Input: dimensioned drawing with shaded views. Units: mm. Origin: part minimum x, y, z. A direction names the side the tool comes from. Give positions to 0.01 mm unless a question says otherwise; leave off trailing zeros. Write each loop counter-clockwise with the first axis right and the second up, starting at its lowest first coordinate (ties: lowest second). Pieces come first, ordered by that corner, then holes. Notation, with made-up numbers: M 41,-34.5 L 53,-34.5 A25 cw 53,-4.5 Z; hole C 40.5,-34 d11. An arc over 180 degrees is marked long. Answer as a JSON object with one key per item and string values.
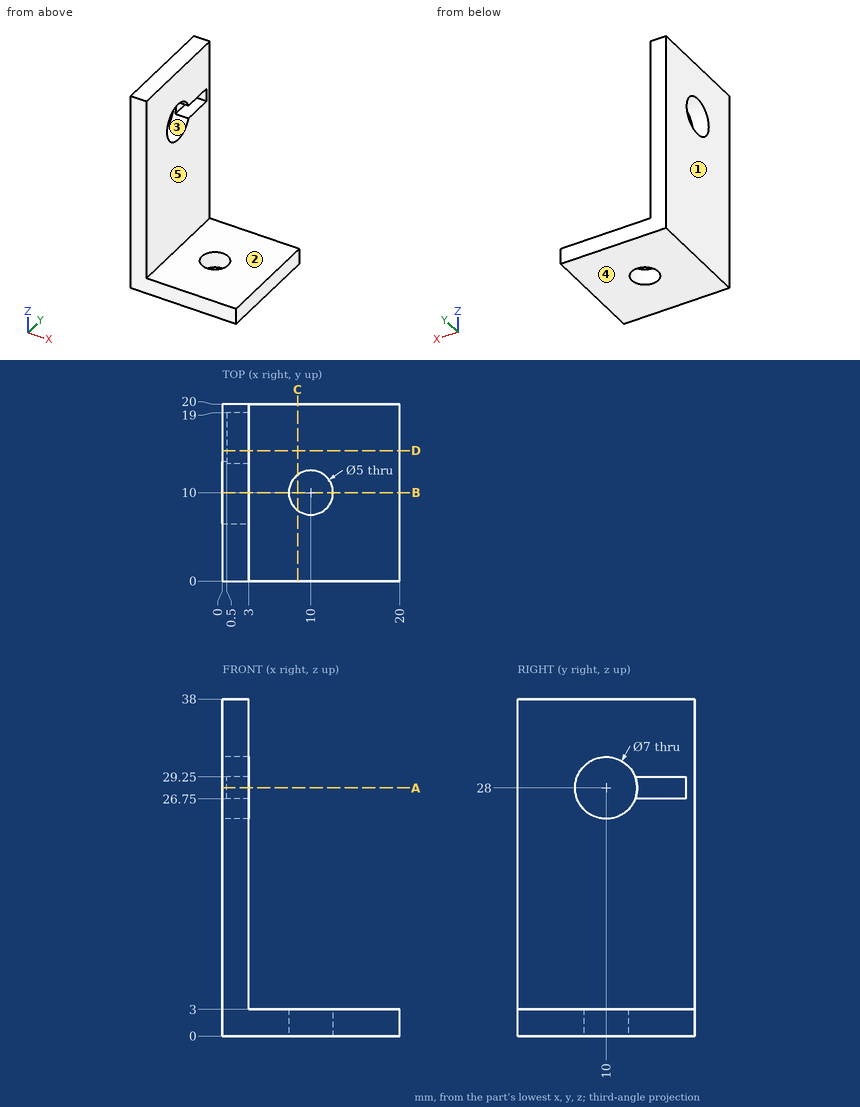
1) Cut plane A-A on z = 28. Return loops of the section in (x, y), and give its area (4 significant figures).
Geometry check:
{"outline": "M 0,0 L 3,0 L 3,6.5 L 0,6.5 Z; M 0,13.5 L 0.5,13.5 L 0.5,19 L 3,19 L 3,20 L 0,20 Z", "area": "25.25 mm2"}
2) Cut plane D-D on y = 14.75. Return loops of the section in (x, z).
Geometry check:
{"outline": "M 0,0 L 20,0 L 20,3 L 3,3 L 3,26.75 L 0.5,26.75 L 0.5,29.25 L 3,29.25 L 3,38 L 0,38 Z"}
3) Line query: line 1 (Y direction, x = 10, z = 0.9); line 2 (Z direction, x = 0.95, y = 10); line 3 (Y direction, x = 0.7, z = 28). Output: solid intervals per line, ascending. Write a range as from..to.
Geometry check:
{"line 1": "y = 0..7.5, 12.5..20", "line 2": "z = 0..24.5, 31.5..38", "line 3": "y = 0..6.5, 19..20"}
4) Cut plane C-C on x = 8.5. Return loops of the section in (y, z).
Geometry check:
{"outline": "M 0,0 L 8,0 L 8,3 L 0,3 Z; M 12,0 L 20,0 L 20,3 L 12,3 Z"}
5) Set-up query: the marked faces 4 and 5. Return all of +Z, -Z, +X, -X, +Y, -Y with unobstructed straight access to the full face (end or side cutting, diameter ignored); none if empty.
Geometry check:
{"face 4": "-Z, +X, -X, +Y, -Y", "face 5": "+Z, +X, +Y, -Y"}
6) Pull-direction query (Z, two-part tool) for the marked faces 1, 2 and 3; classes: pulls with the +Z half, pulls with the -Z half, needs draft (parallel to the pull), parting line crosses it, or undercut.
Geometry check:
{"face 1": "needs draft", "face 2": "pulls with the +Z half", "face 3": "undercut"}
7) Cut plane B-B on y = 10. Return loops of the section in (x, z), and give its area (3 significant figures).
Geometry check:
{"outline": "M 0,0 L 7.5,0 L 7.5,3 L 3,3 L 3,24.5 L 0,24.5 Z; M 0,31.5 L 3,31.5 L 3,38 L 0,38 Z; M 12.5,0 L 20,0 L 20,3 L 12.5,3 Z", "area": "129 mm2"}
8) Contact query for flat-ended pins moving along their axis: P1, Ø5, axis at x = 6, y = 10, coming from the -Z side; P2, Ø1, axis at x = 4, z = 21.5, coming from the +Y side; P3, Ø9, axis at y = 10, z = 28, coming from the +X side; P4, Ø8.5, axis at x = 13.5, y = 14, coming from the +Z side. Output: stop coordinate, or through.
Geometry check:
{"P1": "stops at z = 0", "P2": "passes through", "P3": "stops at x = 3", "P4": "stops at z = 3"}
